The listing builds one solid part. Answer for the finished solid, in the listing's coordinates (mm). Face numbers are marked on the shaded views. Give positions to 0.01 mm unless a question says otherwise; leave off trailing zeros. Order: outer loops, then holes, each group sorted by start corner. A loop starts at its lowest first (then second) coordinate and runs counter-clockwise, first axis right, second up. Notation, with made-up numbers: (-34, 14.25) - (-9, 14.25) arc R17 ccw to (-9, 45.25) - close; hole circle Ø8 at (-36, 37.5). An arc over 180 degrees is marked (long way). Answer as CSV lines item,"result". Start each with the question number.
1. Consider line 1 along Y through (x, z) = (4, 11); line 2 along X through (y, z) = (43.75, 10); line 3 along Y through (x, z) = (-9.5, 21.5). Determine where each line is inside the solid, lowest interval first. Write a range as [from, to].
2. Determine the mould class of the marked faces 1, 2, 3 and 4 for opening direction X: +X half, -X half, draft (parallel to the pull), parting line (faces both ways), or undercut.
3. Section B-B on x = 29 is taken. Give the vertices of the cut face in (y, z).
4. Section D-D on y = 38.75 is taken. Give the vertices of the cut face in (x, z), and give its area (3 significant figures).
5. Flat-ended cylindrical pins translate along their axes: pin 1 (2 mm diameter, centred on x = 12.5, y = 37, fed in from +Z); pin 2 (1 mm diameter, centred on x = 8.5, y = 38.5, fed in from +Z). Find the tip coordinate at first contact, or state that the pin passes through.
6. Section C-C on y = 43.25 is taken. Give the vertices of the cut face in (x, z), and give its area (3 significant figures).
7. Section A-A on z = 7 is taken. Give the vertices of the cut face in (x, y), and give its area (3 significant figures).
from build123d import *

# Parameters (mm, degrees)
F0_W     = 64.703614
F0_H     = 11.739045
F1_DEPTH = 25.4
F2_R     = 5.08
F3_SIZE  = 5.08
F4_T     = -2.54
F5_R     = 5.08


with BuildPart() as f1:
    # F0 (on Top) → F1 (new body)
    with BuildSketch(Plane.XY):
        with Locations((7.69186, 40.92604)):
            Rectangle(F0_W, F0_H)
    extrude(amount=F1_DEPTH)

    # F2
    f2_edges = [f1.edges().sort_by_distance(p)[0] for p in [
        (7.69186, 35.056517, 25.4),
    ]]
    fillet(f2_edges, radius=F2_R)

    # F3
    f3_edges = [f1.edges().sort_by_distance(p)[0] for p in [
        (7.69186, 46.795562, 25.4),
    ]]
    chamfer(f3_edges, length=F3_SIZE)

    # F4
    f4_openings = [f1.faces().sort_by_distance(p)[0] for p in [
        (7.69186, 40.926039, 0),
    ]]
    offset(amount=F4_T, openings=f4_openings)

    # F5
    f5_edges = [f1.edges().sort_by_distance(p)[0] for p in [
        (40.043667, 35.056517, 10.16),
        (-24.659947, 35.056517, 10.16),
    ]]
    fillet(f5_edges, radius=F5_R)


solid = f1.part
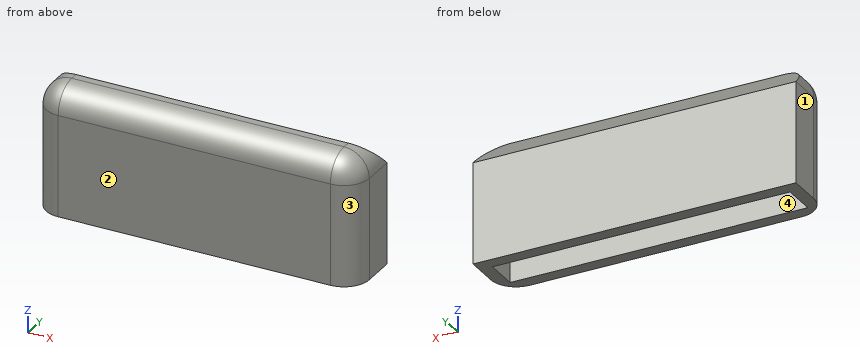
Checks:
1,line 1,"y = [35.06, 37.6], [44.26, 46.8]"
1,line 2,"x = [-24.66, -22.12], [37.5, 40.04]"
1,line 3,"y = [35.2, 37.89], [42.02, 45.62]"
2,face 1,"-X half"
2,face 2,"draft"
2,face 3,"+X half"
2,face 4,"undercut"
3,outline,"(35.06, 0) - (37.6, 0) - (37.6, 20.32) arc R2.54 cw to (40.14, 22.86) - (40.66, 22.86) - (44.26, 19.27) - (44.26, 0) - (46.8, 0) - (46.8, 20.32) - (41.72, 25.4) - (40.14, 25.4) arc R5.08 ccw to (35.06, 20.32) - close"
4,outline,"(-24.47, 0) - (-22.12, 0) - (-22.12, 22.45) - (37.5, 22.45) - (37.5, 0) - (39.85, 0) - (39.85, 20.32) arc R4.89 ccw to (34.96, 25.21) - (-19.58, 25.21) arc R4.89 ccw to (-24.47, 20.32) - close"
4,area,"273 mm²"
5,pin 1,"stops at z = 24.93"
5,pin 2,"stops at z = 25.27"
6,outline,"(-24.66, 0) - (-22.12, 0) - (-22.12, 20.27) - (37.5, 20.27) - (37.5, 0) - (40.04, 0) - (40.04, 20.32) arc R5.08 ccw to (38.6, 23.87) - (-23.22, 23.87) arc R5.08 ccw to (-24.66, 20.32) - close"
6,area,"332 mm²"
7,outline,"(-24.66, 40.14) arc R5.08 ccw to (-19.58, 35.06) - (34.96, 35.06) arc R5.08 ccw to (40.04, 40.14) - (40.04, 46.8) - (-24.66, 46.8) - close; hole (-22.12, 37.6) - (37.5, 37.6) - (37.5, 44.26) - (-22.12, 44.26) - close"
7,area,"351 mm²"
